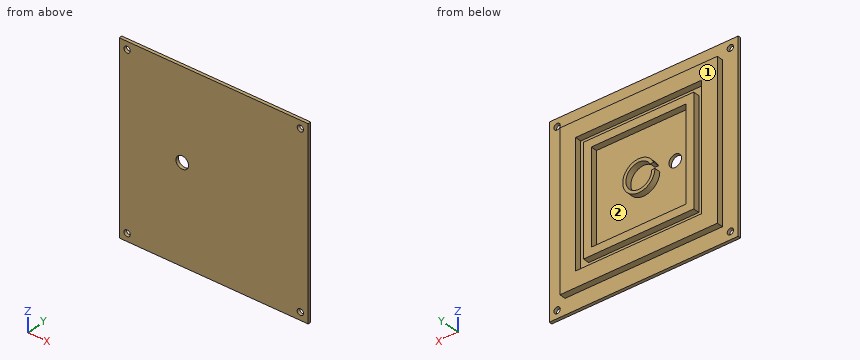
from build123d import *

# Parameters (mm, degrees)
SKETCH1_W           = 152.4
SKETCH1_H           = 152.4
BOSS_EXTRUDE1_DEPTH = 2.54
SKETCH2_W           = 127
SKETCH2_H           = 127
BOSS_EXTRUDE3_DEPTH = 5.08
SKETCH3_W           = 101.6
SKETCH3_H           = 101.6
CUT_EXTRUDE2_DEPTH  = 5.08
SKETCH5_W           = 88.9
SKETCH5_H           = 88.9
BOSS_EXTRUDE4_DEPTH = 5.08
SKETCH6_W           = 76.2
SKETCH6_H           = 76.2
CUT_EXTRUDE3_DEPTH  = 5.08
BOSS_EXTRUDE5_DEPTH = 2.794
SKETCH8_R           = 5.08
CUT_EXTRUDE4_DEPTH  = 3.54
SKETCH9_R           = 2.54
CUT_EXTRUDE5_DEPTH  = 3.54
BOSS_EXTRUDE6_DEPTH = 4.9276


with BuildPart() as part:
    # Sketch1 → Boss-Extrude1 (new body)
    with BuildSketch(Plane(origin=(0, 0, 0), x_dir=(1, 0, 0), z_dir=(0, 1, 0))):
        Rectangle(SKETCH1_W, SKETCH1_H)
    extrude(amount=-BOSS_EXTRUDE1_DEPTH)

    # Sketch2 → Boss-Extrude3 (add)
    with BuildSketch(Plane(origin=(0, 0, 0), x_dir=(1, 0, 0), z_dir=(0, 1, 0))):
        Rectangle(SKETCH2_W, SKETCH2_H)
    extrude(amount=BOSS_EXTRUDE3_DEPTH)

    # Sketch3 → Cut-Extrude2 (cut)
    with BuildSketch(Plane(origin=(0, 5.08, 0), x_dir=(1, 0, 0), z_dir=(0, 1, 0))):
        Rectangle(SKETCH3_W, SKETCH3_H)
    extrude(amount=-CUT_EXTRUDE2_DEPTH, mode=Mode.SUBTRACT)

    # Sketch5 → Boss-Extrude4 (add)
    with BuildSketch(Plane(origin=(0, 0, 0), x_dir=(1, 0, 0), z_dir=(0, 1, 0))):
        Rectangle(SKETCH5_W, SKETCH5_H)
    extrude(amount=BOSS_EXTRUDE4_DEPTH)

    # Sketch6 → Cut-Extrude3 (cut)
    with BuildSketch(Plane(origin=(0, 5.08, 0), x_dir=(1, 0, 0), z_dir=(0, 1, 0))):
        Rectangle(SKETCH6_W, SKETCH6_H)
    extrude(amount=-CUT_EXTRUDE3_DEPTH, mode=Mode.SUBTRACT)

    # Sketch7 → Boss-Extrude5 (add)
    with BuildSketch(Plane(origin=(0, 0, 0), x_dir=(1, 0, 0), z_dir=(0, 1, 0))):
        with BuildLine():
            Line((-10.414, 0), (-12.954, 0))
            ThreePointArc((-12.954, 0), (12.691940102, 2.592445263), (-11.916363371, -5.08))
            Line((-11.916363371, -5.08), (-9.090929325, -5.08))
            ThreePointArc((-9.090929325, -5.08), (10.077805664, 2.624734082), (-10.414, 0))
        make_face()
    extrude(amount=BOSS_EXTRUDE5_DEPTH)

    # Sketch8 → Cut-Extrude4 (cut, through all)
    with BuildSketch(Plane(origin=(0, 0, 0), x_dir=(1, 0, 0), z_dir=(0, 1, 0))):
        with Locations((-25.4, -3.048)):
            Circle(SKETCH8_R)
    extrude(amount=-CUT_EXTRUDE4_DEPTH, mode=Mode.SUBTRACT)

    # Sketch9 → Cut-Extrude5 (cut, through all)
    with BuildSketch(Plane(origin=(0, 0, 0), x_dir=(1, 0, 0), z_dir=(0, 1, 0))):
        with Locations((-69.85, -69.85)):
            Circle(SKETCH9_R)
        with Locations((69.85, -69.85)):
            Circle(SKETCH9_R)
        with Locations((69.85, 69.85)):
            Circle(SKETCH9_R)
        with Locations((-69.85, 69.85)):
            Circle(SKETCH9_R)
    extrude(amount=-CUT_EXTRUDE5_DEPTH, mode=Mode.SUBTRACT)

    # Sketch7<2> → Boss-Extrude6 (add)
    with BuildSketch(Plane(origin=(0, 0, 0), x_dir=(1, 0, 0), z_dir=(0, 1, 0))):
        with BuildLine():
            Line((-10.414, 0), (-12.954, 0))
            ThreePointArc((-12.954, 0), (12.691940102, 2.592445263), (-11.916363371, -5.08))
            Line((-11.916363371, -5.08), (-9.090929325, -5.08))
            ThreePointArc((-9.090929325, -5.08), (10.077805664, 2.624734082), (-10.414, 0))
        make_face()
    extrude(amount=BOSS_EXTRUDE6_DEPTH)


solid = part.part
Geometry check sheet. Reference: the model listing, model coordinates, mm. Face numbers are marked on the shaded views. Round coordinates to 2 decimals unless told otherwise and drop trailing zeros. Write each loop counter-clockwise with the first axis right and the second up, starting at its lowest first coordinate (ties: lowest second). Pieces come first, ordered by that corner, then holes. Notation, with made-up numbers: (51, 70.5) -> (88, 70.5) arc R19 cw to (88, 101.5) -> close; hole circle Ø7 at (-10.5, 64.5). An arc over 180 degrees is marked (long way). One line per item, written item: value. Start each with the question number.
(1) Draft check along Z on the marked faces 1 and 2. Enter one of: +Z half, -Z half, draft (parallel to the pull), parting line (faces both ways), or undercut.
(2) Cross-section at A-A, the plane z = -69.85. Record the cut outline in (x, y).
(3) Cross-section at D-D, the plane x = -25.4. Record the cut outline in (y, z).
(4) Cross-section at C-C, the plane x = 69.85. Record the cut outline in (y, z).
(5) Go/stop test with flat-tipped pins: pin 1 Ø4 at (x, y) = (-7.5, 2.5) entering from -Z; pin 2 Ø2.5 at (x, y) = (-10.5, 2) entering from +Z; pin 3 Ø1.5 at (y, z) = (2, 1.5) entering from -X; pin 4 Ø4 at (x, z) = (69.85, -69.85) entering from +Y. Record where each tip stops, or that it passes through.
(6) Scan lines: line 1 (Z direction, x = -28.5, y = 1.5); line 2 (X direction, y = 4.5, z = -40.5). Record each from-to range of solid material in increasing order. Write a range as [from, to].
(7) Cross-section at B-B, the plane x = 0. Record the cut outline in (y, z), and give its area (3 significant figures).
Answer:
1. face 1: draft
1. face 2: undercut
2. outline: (-76.2, -2.54) -> (-72.39, -2.54) -> (-72.39, 0) -> (-76.2, 0) -> close; (-67.31, -2.54) -> (67.31, -2.54) -> (67.31, 0) -> (-67.31, 0) -> close; (72.39, -2.54) -> (76.2, -2.54) -> (76.2, 0) -> (72.39, 0) -> close
3. outline: (-2.54, -76.2) -> (0, -76.2) -> (0, -63.5) -> (5.08, -63.5) -> (5.08, -50.8) -> (0, -50.8) -> (0, -44.45) -> (5.08, -44.45) -> (5.08, -38.1) -> (0, -38.1) -> (0, -2.03) -> (-2.54, -2.03) -> close; (-2.54, 8.13) -> (0, 8.13) -> (0, 38.1) -> (5.08, 38.1) -> (5.08, 44.45) -> (0, 44.45) -> (0, 50.8) -> (5.08, 50.8) -> (5.08, 63.5) -> (0, 63.5) -> (0, 76.2) -> (-2.54, 76.2) -> close
4. outline: (-2.54, -76.2) -> (0, -76.2) -> (0, -72.39) -> (-2.54, -72.39) -> close; (-2.54, -67.31) -> (0, -67.31) -> (0, 67.31) -> (-2.54, 67.31) -> close; (-2.54, 72.39) -> (0, 72.39) -> (0, 76.2) -> (-2.54, 76.2) -> close
5. pin 1: z = -63.5
5. pin 2: z = 63.5
5. pin 3: x = -63.5
5. pin 4: through
6. line 1: [-63.5, -50.8], [-44.45, -38.1], [38.1, 44.45], [50.8, 63.5]
6. line 2: [-63.5, -50.8], [-44.45, 44.45], [50.8, 63.5]
7. outline: (-2.54, -76.2) -> (0, -76.2) -> (0, -63.5) -> (5.08, -63.5) -> (5.08, -50.8) -> (0, -50.8) -> (0, -44.45) -> (5.08, -44.45) -> (5.08, -38.1) -> (0, -38.1) -> (0, -12.95) -> (4.93, -12.95) -> (4.93, -10.41) -> (0, -10.41) -> (0, 10.41) -> (4.93, 10.41) -> (4.93, 12.95) -> (0, 12.95) -> (0, 38.1) -> (5.08, 38.1) -> (5.08, 44.45) -> (0, 44.45) -> (0, 50.8) -> (5.08, 50.8) -> (5.08, 63.5) -> (0, 63.5) -> (0, 76.2) -> (-2.54, 76.2) -> close
7. area: 606 mm²
